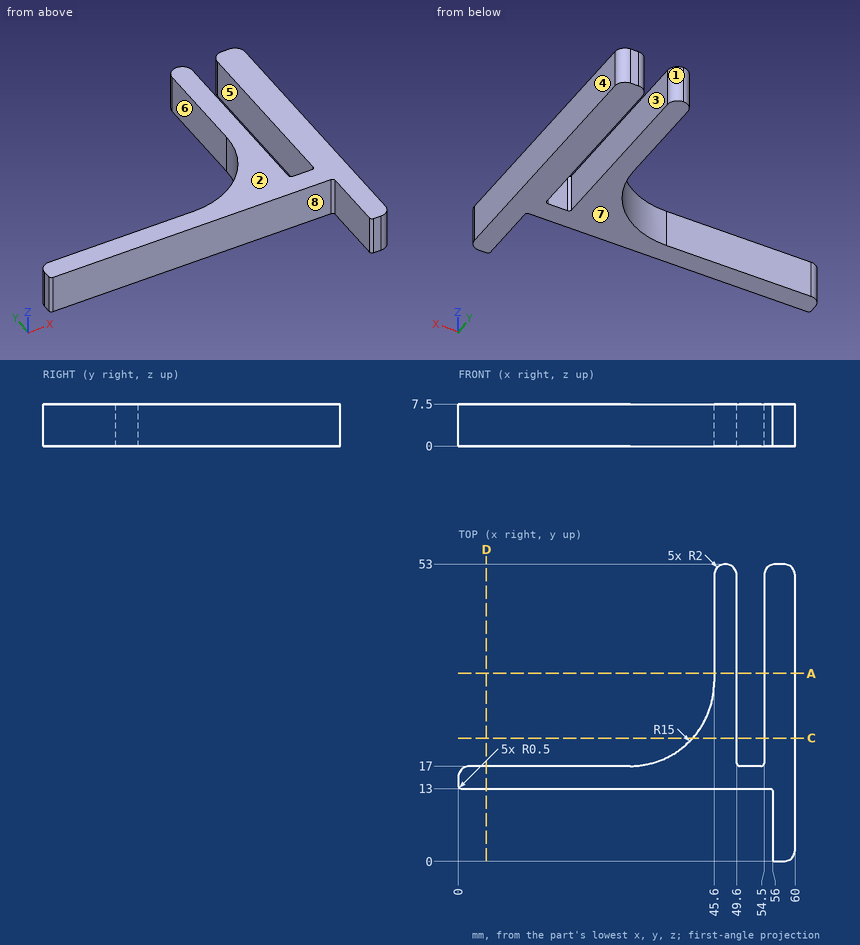
Part print with two shaded views. Sizes in mm from the minimum x, y, z corner. A direction names the side the tool comes from. Coordinates: 2 decimals unless noted, no trailing zeros. Write each loop counter-clockwise with the first axis right and the second up, starting at its lowest first coordinate (ties: lowest second). Pieces come first, ordered by that corner, then holes.
(1) Cut at C-C on y = 22. List the corners of the cut face in (x, z).
(2) Mould opens along X. For the marked faces 1, 2, 3 and 4 say: pulls with the +X half, pulls with the -X half, needs draft (parallel to the pull), parting line crosses it, or undercut.
(3) Cut at A-A on y = 33.5. List the corners of the cut face in (x, z).
(4) 3-axis set-ups, long thin cutter, end or side, ignore diameter. For the marked faces 5, 6, 7 and 8: which of +Z, -Z, +X, -X, +Y, -Y reach the whole face in a straight line?
(5) Cut at D-D on x = 5. List the corners of the cut face in (y, z), and give its area (3 significant figures).
(6) Pin check, flat tips, straight feed: pin 1 Ø5 at (x, y) = (44, 45) entering from +Z; pin 2 Ø4 at (x, z) = (39, 5) entering from -Y; pin 3 Ø2 at (y, z) = (41.5, 5.5) entering from -X; pin 4 Ø4 at (y, z) = (8.5, 4.5) entering from -X. Stop position of each tip, or through.
(7) Drill centre lines: line 1 (X direction, y = 42, z = 6); line 2 (X direction, y = 27.5, z = 3.75); line 3 (Y direction, x = 10, z = 2.5). Where is each one in solid material? Low to high.
Working result:
1. outline: (41.78, 0) - (49.6, 0) - (49.6, 7.5) - (41.78, 7.5) - close; (54.5, 0) - (60, 0) - (60, 7.5) - (54.5, 7.5) - close
2. face 1: undercut
2. face 2: needs draft
2. face 3: undercut
2. face 4: pulls with the +X half
3. outline: (45.6, 0) - (49.6, 0) - (49.6, 7.5) - (45.6, 7.5) - close; (54.5, 0) - (60, 0) - (60, 7.5) - (54.5, 7.5) - close
4. face 5: +Z, -Z, +Y
4. face 6: +Z, -Z, -X, +Y
4. face 7: -Z, +X, -X, +Y, -Y
4. face 8: +Z, -Z, -X, -Y
5. outline: (13, 0) - (17, 0) - (17, 7.5) - (13, 7.5) - close
5. area: 30.0 mm2
6. pin 1: stops at z = 7.5
6. pin 2: stops at y = 13
6. pin 3: stops at x = 45.6
6. pin 4: stops at x = 56
7. line 1: x = 45.6 to 49.6, 54.5 to 60
7. line 2: x = 44.91 to 49.6, 54.5 to 60
7. line 3: y = 13 to 17
